```python
from build123d import *

# Parameters (mm, degrees)
BOX065_W               = 10
BOX065_H               = 94
BOX065_DEPTH           = 4
BOX062_W               = 14
BOX062_H               = 3
BOX062_DEPTH           = 4
BOX061_W               = 14
BOX061_H               = 3
BOX061_DEPTH           = 4
BOX063_W               = 14
BOX063_H               = 3
BOX063_DEPTH           = 4
BOX064_W               = 14
BOX064_H               = 3
BOX064_DEPTH           = 4
SKETCH017_R            = 1.2
SKETCH017_W            = 24
SKETCH017_H            = 13
PAD012_DEPTH           = 140
CYLINDER080_R          = 6
CYLINDER080_DEPTH      = 31
CYLINDER080_ROLL_ANGLE = 90
CYLINDER078_R          = 1.75
CYLINDER078_DEPTH      = 31
CYLINDER078_ROLL_ANGLE = 90
BOX059_W               = 17
BOX059_H               = 77
BOX059_DEPTH           = 49
FILLET018013005_R      = 2
CYLINDER083_R          = 4
CYLINDER083_DEPTH      = 31
CYLINDER083_ROLL_ANGLE = 90
CYLINDER079_R          = 1.75
CYLINDER079_DEPTH      = 31
CYLINDER079_ROLL_ANGLE = 90
BOX058_W               = 8
BOX058_H               = 24
BOX058_DEPTH           = 11
BOX057_W               = 76
BOX057_H               = 76
BOX057_DEPTH           = 66
FILLET018013003_R      = 3.5
BOX060_W               = 80
BOX060_H               = 80
BOX060_DEPTH           = 63
FILLET018013006_R      = 1


with BuildPart() as cubo:
    # Box065 → Box065 (new body)
    with BuildSketch(Plane(origin=(13, -11, 104), x_dir=(1, 0, 0), z_dir=(0, 0, 1))):
        with Locations((5, 47)):
            Rectangle(BOX065_W, BOX065_H)
    extrude(amount=BOX065_DEPTH)


with BuildPart() as cubo009:
    # Box062 → Box062 (new body)
    with BuildSketch(Plane(origin=(11, 75.5, 127), x_dir=(1, 0, 0), z_dir=(0, 0, 1))):
        with Locations((7, 1.5)):
            Rectangle(BOX062_W, BOX062_H)
    extrude(amount=BOX062_DEPTH)


with BuildPart() as cubo008:
    # Box061 → Box061 (new body)
    with BuildSketch(Plane(origin=(11, 75.5, 109), x_dir=(1, 0, 0), z_dir=(0, 0, 1))):
        with Locations((7, 1.5)):
            Rectangle(BOX061_W, BOX061_H)
    extrude(amount=BOX061_DEPTH)


with BuildPart() as cubo010:
    # Box063 → Box063 (new body)
    with BuildSketch(Plane(origin=(11, -6.5, 109), x_dir=(1, 0, 0), z_dir=(0, 0, 1))):
        with Locations((7, 1.5)):
            Rectangle(BOX063_W, BOX063_H)
    extrude(amount=BOX063_DEPTH)


with BuildPart() as cubo011:
    # Box064 → Box064 (new body)
    with BuildSketch(Plane(origin=(11, -6.5, 127), x_dir=(1, 0, 0), z_dir=(0, 0, 1))):
        with Locations((7, 1.5)):
            Rectangle(BOX064_W, BOX064_H)
    extrude(amount=BOX064_DEPTH)


with BuildPart() as pad012:
    # Sketch017 → Pad012 (new body)
    with BuildSketch(Plane(origin=(-0.25, -35, 0), x_dir=(1, 0, 0), z_dir=(0, -1, 0))):
        with Locations((37, 120)):
            Circle(SKETCH017_R)
        with Locations((9.5, 120)):
            Circle(SKETCH017_R)
        with Locations((23.25, 120)):
            Rectangle(SKETCH017_W, SKETCH017_H)
    extrude(amount=-PAD012_DEPTH)


with BuildPart() as cylinder107:
    # Cylinder080 → Cylinder080 (new body)
    with BuildSketch(Plane.XY):
        Circle(CYLINDER080_R)
    extrude(amount=CYLINDER080_DEPTH)


with BuildPart() as cylinder107_1:
    # Cylinder080 roll: moved
    add(cylinder107.part.rotate(Axis((0, 0, 0), (1, 0, 0)), CYLINDER080_ROLL_ANGLE))


with BuildPart() as cylinder107_2:
    # Cylinder080 placement: moved
    add(cylinder107_1.part.moved(Location((-4, 11, 83.5))))


with BuildPart() as cylinder105:
    # Cylinder078 → Cylinder078 (new body)
    with BuildSketch(Plane.XY):
        Circle(CYLINDER078_R)
    extrude(amount=CYLINDER078_DEPTH)


with BuildPart() as cylinder105_1:
    # Cylinder078 roll: moved
    add(cylinder105.part.rotate(Axis((0, 0, 0), (1, 0, 0)), CYLINDER078_ROLL_ANGLE))


with BuildPart() as cylinder105_2:
    # Cylinder078 placement: moved
    add(cylinder105_1.part.moved(Location((-8.5, 11, 71.5))))


with BuildPart() as fillet018013005:
    # Box059 → Box059 (new body)
    with BuildSketch(Plane(origin=(-14, -2.5, 75), x_dir=(1, 0, 0), z_dir=(0, 0, 1))):
        with Locations((8.5, 38.5)):
            Rectangle(BOX059_W, BOX059_H)
    extrude(amount=BOX059_DEPTH)

    # Fillet018013005
    fillet018013005_edges = [fillet018013005.edges().sort_by_distance(p)[0] for p in [
        (-14, -2.5, 99.5),
        (-14, 36, 124),
        (-14, 74.5, 99.5),
        (-14, 36, 75),
        (3, -2.5, 99.5),
        (3, 36, 124),
        (3, 74.5, 99.5),
        (3, 36, 75),
        (-5.5, -2.5, 75),
        (-5.5, -2.5, 124),
        (-5.5, 74.5, 75),
        (-5.5, 74.5, 124),
    ]]
    fillet(fillet018013005_edges, radius=FILLET018013005_R)


with BuildPart() as cylinder108:
    # Cylinder083 → Cylinder083 (new body)
    with BuildSketch(Plane.XY):
        Circle(CYLINDER083_R)
    extrude(amount=CYLINDER083_DEPTH)


with BuildPart() as cylinder108_1:
    # Cylinder083 roll: moved
    add(cylinder108.part.rotate(Axis((0, 0, 0), (1, 0, 0)), CYLINDER083_ROLL_ANGLE))


with BuildPart() as cylinder108_2:
    # Cylinder083 placement: moved
    add(cylinder108_1.part.moved(Location((-7, 80, 89.6))))


with BuildPart() as cylinder106:
    # Cylinder079 → Cylinder079 (new body)
    with BuildSketch(Plane.XY):
        Circle(CYLINDER079_R)
    extrude(amount=CYLINDER079_DEPTH)


with BuildPart() as cylinder106_1:
    # Cylinder079 roll: moved
    add(cylinder106.part.rotate(Axis((0, 0, 0), (1, 0, 0)), CYLINDER079_ROLL_ANGLE))


with BuildPart() as cylinder106_2:
    # Cylinder079 placement: moved
    add(cylinder106_1.part.moved(Location((-8.5, 80, 71.5))))


with BuildPart() as fusion061:
    # Box058 → Box058 (new body)
    with BuildSketch(Plane(origin=(-13.5, -13, 95), x_dir=(1, 0, 0), z_dir=(0, 0, 1))):
        with Locations((4, 12)):
            Rectangle(BOX058_W, BOX058_H)
    extrude(amount=BOX058_DEPTH)

    # Fusion061: union Cylinder107, Cylinder105, Fillet018013005, Cylinder108, Cylinder106
    add(cylinder107_2.part)
    add(cylinder105_2.part)
    add(fillet018013005.part)
    add(cylinder108_2.part)
    add(cylinder106_2.part)


with BuildPart() as fillet018013003:
    # Box057 → Box057 (new body)
    with BuildSketch(Plane(origin=(-21, -2, 87), x_dir=(1, 0, 0), z_dir=(0, 0, 1))):
        with Locations((38, 38)):
            Rectangle(BOX057_W, BOX057_H)
    extrude(amount=BOX057_DEPTH)

    # Fillet018013003
    fillet018013003_edges = [fillet018013003.edges().sort_by_distance(p)[0] for p in [
        (-21, -2, 120),
        (-21, 36, 153),
        (-21, 74, 120),
        (55, -2, 120),
        (55, 36, 153),
        (55, 74, 120),
        (17, -2, 153),
        (17, 74, 153),
    ]]
    fillet(fillet018013003_edges, radius=FILLET018013003_R)


with BuildPart() as fillet018013003_1:
    # Fillet018013003 placement: moved
    add(fillet018013003.part.moved(Location((0, 0, -24))))


with BuildPart() as obj1:
    # Box060 → Box060 (new body)
    with BuildSketch(Plane(origin=(-23, -4, 68), x_dir=(1, 0, 0), z_dir=(0, 0, 1))):
        with Locations((40, 40)):
            Rectangle(BOX060_W, BOX060_H)
    extrude(amount=BOX060_DEPTH)

    # Cut103: cut Fillet018013003
    add(fillet018013003_1.part, mode=Mode.SUBTRACT)

    # Cut104: cut Fusion061
    add(fusion061.part, mode=Mode.SUBTRACT)

    # Cut105: cut Pad012
    add(pad012.part, mode=Mode.SUBTRACT)

    # Fusion062: union Cubo009, Cubo008, Cubo010, Cubo011
    add(cubo009.part)
    add(cubo008.part)
    add(cubo010.part)
    add(cubo011.part)

    # Fillet018013006
    fillet018013006_edges = [obj1.edges().sort_by_distance(p)[0] for p in [
        (25, -6.5, 129),
        (11, -6.5, 129),
        (11, -6.5, 111),
        (25, -6.5, 111),
        (25, 78.5, 129),
        (11, 78.5, 129),
        (25, 78.5, 111),
        (11, 78.5, 111),
    ]]
    fillet(fillet018013006_edges, radius=FILLET018013006_R)

    # Cut107: cut Cubo
    add(cubo.part, mode=Mode.SUBTRACT)


solid = obj1.part
```
Model file for the job. Use its own axes, mm. A direction names the side the tool comes from. Round coordinates to 2 decimals unless told otherwise and drop trailing zeros. Order: outer loops, then holes, each group sorted by start corner. A loop starts at its lowest first (then second) coordinate and runs counter-clockwise, first axis right, second up. Notation, with made-up numbers: (-22, 76.5) -> (34, 76.5) arc R18 cw to (34, 88.5) -> close; hole circle Ø10 at (30.5, 57.25). An arc over 180 degrees is marked (long way). Use one line per item in the form item = value.
Item 1: Tool access for faces 1 (the face through (-7.521, 75.261, 93.566)), 2 (the face through (23, 75, 113.5)), 3 (the face through (-6, 74.5, 99)), 4 (the face through (55, 36, 96)): list every direction of +Z, -Z, +X, -X, +Y, -Y with a clear straight run to the whole face (end or side of a thin tool).
Returned:
face_1 = +Y
face_2 = +Y, -Y
face_3 = none
face_4 = -Z
Item 2: Cut at C-C, the plane y = 41. Write the cut outline in (x, z), and give its area (3 significant figures).
Returned:
outline = (-23, 68) -> (-21, 68) -> (-21, 125.5) arc R3.5 cw to (-17.5, 129) -> (51.5, 129) arc R3.5 cw to (55, 125.5) -> (55, 68) -> (57, 68) -> (57, 131) -> (-23, 131) -> close
area = 409 mm^2
Item 3: Cut at B-B, the plane z = 116. Write the cut outline in (x, y).
Returned:
outline = (-23, -4) -> (11, -4) -> (11, -2) -> (2.32, -2) arc R2 cw to (1, -2.5) -> (-12, -2.5) arc R2 cw to (-13.32, -2) -> (-17.5, -2) arc R3.5 cw to (-21, 1.5) -> (-21, 70.5) arc R3.5 cw to (-17.5, 74) -> (-13.32, 74) arc R2 cw to (-12, 74.5) -> (1, 74.5) arc R2 cw to (2.32, 74) -> (11, 74) -> (11, 76) -> (-23, 76) -> close; (35, -4) -> (57, -4) -> (57, 76) -> (35, 76) -> (35, 74) -> (51.5, 74) arc R3.5 cw to (55, 70.5) -> (55, 1.5) arc R3.5 cw to (51.5, -2) -> (35, -2) -> close
Item 4: Cut at D-D, the plane z = 71.5. Write the cut outline in (x, y).
Returned:
outline = (-23, -4) -> (-10.25, -4) -> (-10.25, -2) -> (-17.5, -2) arc R3.5 cw to (-21, 1.5) -> (-21, 70.5) arc R3.5 cw to (-17.5, 74) -> (-10.25, 74) -> (-10.25, 76) -> (-23, 76) -> close; (-6.75, -4) -> (57, -4) -> (57, 76) -> (-6.75, 76) -> (-6.75, 74) -> (51.5, 74) arc R3.5 cw to (55, 70.5) -> (55, 1.5) arc R3.5 cw to (51.5, -2) -> (-6.75, -2) -> close
Item 5: Cut at A-A, the plane x = 36.75. Write the cut outline in (y, z), and give its area (3 significant figures).
Returned:
outline = (-4, 68) -> (-2, 68) -> (-2, 118.8) -> (-4, 118.8) -> close; (-4, 121.2) -> (-2, 121.2) -> (-2, 125.5) arc R3.5 cw to (1.5, 129) -> (70.5, 129) arc R3.5 cw to (74, 125.5) -> (74, 121.2) -> (76, 121.2) -> (76, 131) -> (-4, 131) -> close; (74, 68) -> (76, 68) -> (76, 118.8) -> (74, 118.8) -> close
area = 400 mm^2
Item 6: Flat gauge pins, fed straight in: pin 1 Ø2 at (x, y) = (10.5, 41.5) entering from -Z; pin 2 Ø17 at (x, z) = (6.5, 92) entering from +Y; pin 3 Ø8 at (x, z) = (12.5, 103) entering from -Y. Where does each tip first touch, or does it go through?
Returned:
pin_1 = 129
pin_2 = 76
pin_3 = -4
Item 7: Pull direction X, two halves, no side cores. Call faces 5 (the face through (57, 35, 99)), 6 (the face through (-20, -0.95, 97.15)), 7 (the face through (18, -5, 127)): released by +X, released by -X, zero draft, split by the parting line, or undercut.
Returned:
face_5 = released by +X
face_6 = undercut
face_7 = zero draft
Item 8: Drill centre lines: line 1 (X direction, y = 74.65, z = 120); line 2 (X direction, y = 19.5, z = 121); line 3 (X direction, y = -2.75, z = 83.5). Where is each one in solid material? Low to high.
Returned:
line_1 = -23 to 8.05, 10.45 to 11, 35 to 35.55, 37.95 to 57
line_2 = -23 to -21, 55 to 57
line_3 = -23 to -10, 2 to 57
